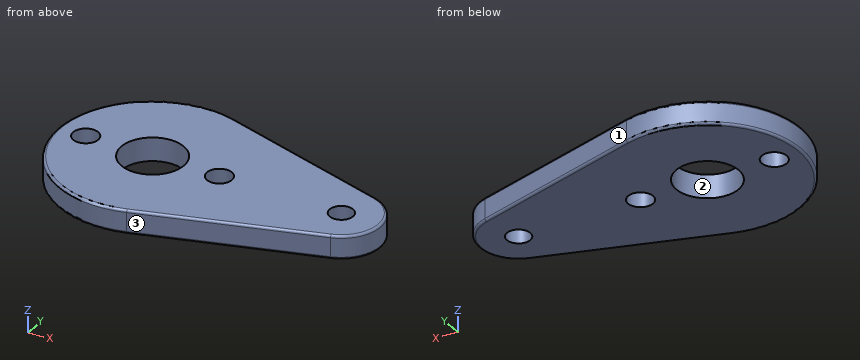
```python
from build123d import *

# Parameters (mm, degrees)
ESQUISSE1_R        = 4
ESQUISSE1_R_2      = 1.5
ESQUISSE1_R_3      = 1.6
BOSS_EXTRU_1_DEPTH = 3
CONG_2_R           = 0.3


with BuildPart() as part:
    # Esquisse1 → Boss.-Extru.1 (new body)
    with BuildSketch(Plane.XY):
        with BuildLine():
            Line((3.5, 11.478240283), (25.458333333, 4.782600118))
            ThreePointArc((25.458333333, 4.782600118), (29, 0), (25.458333333, -4.782600118))
            Line((25.458333333, -4.782600118), (3.5, -11.478240283))
            ThreePointArc((3.5, -11.478240283), (-12, 0), (3.5, 11.478240283))
        make_face()
        Circle(ESQUISSE1_R, mode=Mode.SUBTRACT)
        with Locations((24, 0)):
            Circle(ESQUISSE1_R_2, mode=Mode.SUBTRACT)
        with Locations((-8.5, 0)):
            Circle(ESQUISSE1_R_3, mode=Mode.SUBTRACT)
        with Locations(Location((8.5, 0, 0), (0, 0, 180))):
            Circle(ESQUISSE1_R_3, mode=Mode.SUBTRACT)
    extrude(amount=BOSS_EXTRU_1_DEPTH)

    # Congé2
    cong_2_edges = [part.edges().sort_by_distance(p)[0] for p in [
        (29, 0, 3),
        (14.479166667, 8.130420201, 3),
        (-12, 0, 3),
        (14.479166667, 8.130420201, 0),
        (29, 0, 0),
        (14.479166667, -8.130420201, 0),
        (-12, 0, 0),
        (14.479166667, -8.130420201, 3),
    ]]
    fillet(cong_2_edges, radius=CONG_2_R)


solid = part.part
```
Geometry: final body of the model. Coordinates: model frame, mm. Face numbers are marked on the shaded views. Round coordinates to 2 decimals unless told otherwise and drop trailing zeros. Write each loop counter-clockwise with the first axis right and the second up, starting at its lowest first coordinate (ties: lowest second). Pieces come first, ordered by that corner, then holes. Notation, with made-up numbers: (60.5, 24.5) -> (105.5, 24.5) arc R28 ccw to (105.5, 53.5) -> close; hole circle Ø7 at (-26.75, 45.25). An arc over 180 degrees is marked (long way). Return JSON: item names as keys, results as strings.
Q1. First-contact query: pin 1 Ø1 at (x, z) = (12, 1.5) entering from -Y; pin 2 Ø1.5 at (x, z) = (7, 2.5) entering from +Y. Flat tips, straight axial feed; report the tip coordinate or a pass-through.
From the geometry:
{"pin 1": "y = -9.04", "pin 2": "y = 10.64"}
Q2. Mould query, pull axis Y, two halves, no side actions, for the marked faces 1, 2 and 3. Classes: +Y half, -Y half, draft (parallel to the pull), parting line (faces both ways), or undercut.
From the geometry:
{"face 1": "+Y half", "face 2": "undercut", "face 3": "-Y half"}
Q3. Section A-A on z = 1.75. Return the cut outline in (x, y).
From the geometry:
{"outline": "(3.5, -11.48) -> (25.46, -4.78) arc R5 ccw to (25.46, 4.78) -> (3.5, 11.48) arc R12 ccw (long way) to start; hole circle Ø3.2 at (-8.5, 0); hole circle Ø8 at (0, 0); hole circle Ø3.2 at (8.5, 0); hole circle Ø3 at (24, 0)"}
Q4. Ray query, line 1 (Y direction, x = 24, z = 2.3); line 2 (X direction, y = -1.25, z = 0.9); line 3 (X direction, y = 2.25, z = 2.7). Return the intervals inside material, ascending.
From the geometry:
{"line 1": "-5.23 to -1.5, 1.5 to 5.23", "line 2": "-11.93 to -9.5, -7.5 to -3.8, 3.8 to 7.5, 9.5 to 23.17, 24.83 to 28.84", "line 3": "-11.79 to -3.31, 3.31 to 28.47"}
